```python
from build123d import *

# Parameters (mm, degrees)
EXTRUDE_1_DEPTH           = 20
FILLET_1_R                = 5
SKETCH_2_R                = 8
CUT_EXTRUDE_1_DEPTH       = 5
SKETCH_3_R                = 6
CUT_EXTRUDE_2_DEPTH       = 1
CUT_EXTRUDE_3_DEPTH       = 5
CUT_EXTRUDE_4_DEPTH       = 5
SKETCH_6_R                = 0.625
CUT_EXTRUDE_5_DEPTH       = 4
SKETCH_7_W                = 27
SKETCH_7_H                = 5
CUT_EXTRUDE_6_DEPTH       = 7
SKETCH_8_R                = 1.45
CUT_EXTRUDE_7_DEPTH       = 12
CUT_EXTRUDE_8_DEPTH       = 43.204857647
SKETCH_10_W               = 7.5
SKETCH_10_H               = 8.2
CUT_EXTRUDE_9_DEPTH       = 35.875672037
CUT_EXTRUDE_10_DEPTH      = 40.749968553
CUT_EXTRUDE_10_DEPTH_BACK = 40.749968553
SKETCH_11_R               = 1.455


with BuildPart() as part:
    # Эскиз1 → Бобышка-Вытянуть1 (new body)
    with BuildSketch(Plane(origin=(0, 0, 0), x_dir=(1, 0, 0), z_dir=(0, 1, 0))):
        Polygon((-13, 27.5), (-13, 0), (13, 0), (13, 27.5), (25, 27.5), (25, -7.5), (-25, -7.5), (-25, 27.5), align=None)
    extrude(amount=EXTRUDE_1_DEPTH)

    # Скругление1
    fillet_1_edges = [part.edges().sort_by_distance(p)[0] for p in [
        (19, 0, -27.5),
        (25, 10, -27.5),
        (-25, 10, -27.5),
        (-19, 20, -27.5),
        (-25, 20, -10),
        (25, 20, -10),
        (19, 20, -27.5),
        (25, 0, -10),
        (-25, 0, -10),
        (-19, 0, -27.5),
    ]]
    fillet(fillet_1_edges, radius=FILLET_1_R)

    # Эскиз2 → Вырез-Вытянуть1 (cut)
    with BuildSketch(Plane.ZY.offset(-13)):
        with Locations((-17.5, 10)):
            Circle(SKETCH_2_R)
    extrude(amount=-CUT_EXTRUDE_1_DEPTH, mode=Mode.SUBTRACT)

    # Эскиз3 → Вырез-Вытянуть2 (cut)
    with BuildSketch(Plane.ZY.offset(-18)):
        with Locations((-17.5, 10)):
            Circle(SKETCH_3_R)
    extrude(amount=-CUT_EXTRUDE_2_DEPTH, mode=Mode.SUBTRACT)

    # Эскиз4 → Вырез-Вытянуть3 (cut)
    with BuildSketch(Plane(origin=(-13, 0, 0), x_dir=(0, 0, -1), z_dir=(1, 0, 0))):
        with BuildLine():
            Line((13.195, 19.30212207), (2.9, 14.537620522))
            ThreePointArc((2.9, 14.537620522), (0, 10), (2.9, 5.462379478))
            Line((2.9, 5.462379478), (13.195, 0.69787793))
            ThreePointArc((13.195, 0.69787793), (27.75, 10), (13.195, 19.30212207))
        make_face()
    extrude(amount=-CUT_EXTRUDE_3_DEPTH, mode=Mode.SUBTRACT)

    # Эскиз5 → Вырез-Вытянуть4 (cut)
    with BuildSketch(Plane(origin=(-18, 0, 0), x_dir=(0, 0, -1), z_dir=(1, 0, 0))):
        with BuildLine():
            Line((19.4, 15.812916652), (19.4, 16.49838717))
            ThreePointArc((19.4, 16.49838717), (17.499999842, 18.39838717), (15.6, 16.498386854))
            Line((15.6, 16.498386854), (15.6, 15.665366642))
            ThreePointArc((15.6, 15.665366642), (15.094249889, 14.335999398), (13.832782732, 13.678959785))
            Line((13.832782732, 13.678959785), (1.932299859, 12.284367885))
            ThreePointArc((1.932299859, 12.284367885), (-0.1, 10), (1.932299859, 7.715632115))
            Line((1.932299859, 7.715632115), (13.832782732, 6.321040215))
            ThreePointArc((13.832782732, 6.321040215), (15.094249889, 5.664000602), (15.6, 4.334633358))
            Line((15.6, 4.334633358), (15.6, 3.501613146))
            ThreePointArc((15.6, 3.501613146), (17.5, 1.601613146), (19.4, 3.501613146))
            Line((19.4, 3.501613146), (19.4, 4.187083665))
            ThreePointArc((19.4, 4.187083665), (19.635266181, 5.128207436), (20.285714286, 5.847916677))
            ThreePointArc((20.285714286, 5.847916677), (22.5, 10), (20.285714286, 14.152083323))
            ThreePointArc((20.285714286, 14.152083323), (19.635266107, 14.871792704), (19.4, 15.812916652))
        make_face()
    extrude(amount=-CUT_EXTRUDE_4_DEPTH, mode=Mode.SUBTRACT)

    # Эскиз6 → Вырез-Вытянуть5 (cut)
    with BuildSketch(Plane(origin=(-23, 0, 0), x_dir=(0, 0, -1), z_dir=(1, 0, 0))):
        with Locations((2.278018202, 10)):
            Circle(SKETCH_6_R)
        with Locations((6.311115384, 10)):
            Circle(SKETCH_6_R)
        with Locations((10.428235425, 10)):
            Circle(SKETCH_6_R)
        with Locations((17.5, 14.907931149)):
            Circle(SKETCH_6_R)
        with Locations((17.5, 16.848859168)):
            Circle(SKETCH_6_R)
        with Locations((17.5, 5.082068851)):
            Circle(SKETCH_6_R)
        with Locations((17.5, 3.141140832)):
            Circle(SKETCH_6_R)
    extrude(amount=-CUT_EXTRUDE_5_DEPTH, mode=Mode.SUBTRACT)

    # Эскиз7 → Вырез-Вытянуть6 (cut)
    with BuildSketch(Plane.XY.offset(7.5)):
        with Locations((0, 17.5)):
            Rectangle(SKETCH_7_W, SKETCH_7_H)
        with Locations((0, 2.5)):
            Rectangle(SKETCH_7_W, SKETCH_7_H)
    extrude(amount=-CUT_EXTRUDE_6_DEPTH, mode=Mode.SUBTRACT)

    # Эскиз8 → Вырез-Вытянуть7 (cut)
    with BuildSketch(Plane(origin=(0, 15, 0), x_dir=(1, 0, 0), z_dir=(0, 1, 0))):
        with Locations(Location((-8.5, -4, 0), (0, 0, 270))):
            Circle(SKETCH_8_R)
        with Locations(Location((8.5, -4, 0), (0, 0, 270))):
            Circle(SKETCH_8_R)
    extrude(amount=-CUT_EXTRUDE_7_DEPTH, mode=Mode.SUBTRACT)

    # Эскиз9 → Вырез-Вытянуть8 (cut, through all)
    with BuildSketch(Plane.XZ):
        Polygon((13, 0), (17.25, 0), (17.25, 7.5), (-36.683406806, 12.049060371), (-29.579948377, -33.351304372), (-5.181112902, -33.351304372), (8.202214573, -2.26080516), align=None)
    extrude(amount=-CUT_EXTRUDE_8_DEPTH, mode=Mode.SUBTRACT)

    # Эскиз10 → Вырез-Вытянуть9 (cut, through all)
    with BuildSketch(Plane.ZY.offset(-17.25)):
        with Locations((3.75, 10)):
            Rectangle(SKETCH_10_W, SKETCH_10_H)
    extrude(amount=-CUT_EXTRUDE_9_DEPTH, mode=Mode.SUBTRACT)

    # Эскиз11 → Вырез-Вытянуть10 (cut, two sides: drawn at the far end of the back side and taken through both)
    with BuildSketch(Plane(origin=(0, 5.9, 0), x_dir=(1, 0, 0), z_dir=(0, 1, 0)).offset(-CUT_EXTRUDE_10_DEPTH_BACK)):
        with Locations(Location((21, -3.75, 0), (0, 0, 270))):
            Circle(SKETCH_11_R)
    extrude(amount=CUT_EXTRUDE_10_DEPTH + CUT_EXTRUDE_10_DEPTH_BACK, mode=Mode.SUBTRACT)


solid = part.part
```
Input: part model. Units: mm. Frame: model coordinates. A direction names the side the tool comes from. Round coordinates to 2 decimals unless told otherwise and drop trailing zeros. Order: outer loops, then holes, each group sorted by start corner. A loop starts at its lowest first (then second) coordinate and runs counter-clockwise, first axis right, second up. Notation, with made-up numbers: (0, 86.5) - (37, 86.5) arc R10 ccw to (37, 93.5) - close; hole circle Ø9 at (-1, 45). An arc over 180 degrees is marked (long way). Answer in a Markdown table with one row per item.
Item 1: Section query D-D (z = -17.5). Return the cut outline in (x, y).
Model answer:
| item | result |
|---|---|
| outline | (13, 0) - (20, 0) arc R5 ccw to (25, 5) - (25, 15) arc R5 ccw to (20, 20) - (13, 20) - (13, 18) - (18, 18) - (18, 16) - (19, 16) - (19, 4) - (18, 4) - (18, 2) - (13, 2) - close |
Item 2: Reachability of faces 1 (the flat face through (21, 5.9, 2)), 2 (the flat face through (18, 10, 0)), 3 (the flat face through (17.25, 3, 4)) from +Z, -Z, +X, -X, +Y, -Y: full face, straight path, thin tool, end or side. Return the list, or none.
Model answer:
| item | result |
|---|---|
| face 1 | +Z, +X, -X |
| face 2 | +Z, -X |
| face 3 | +Z, -X, +Y, -Y |
Item 3: Mould query, pull axis X, two halves, no side actions, for faces 4 (the cylindrical face through (19.58, 17.01, 3.43)), 5 (the cylindrical face through (16.55, 1.5, -26.07)), 6 (the flat face through (18, 16, -16)), 7 (the cylindrical face through (19.58, 2.91, 3.43)). Classes: released by +X, released by -X, zero draft, split by the parting line, or undercut.
Model answer:
| item | result |
|---|---|
| face 4 | undercut |
| face 5 | zero draft |
| face 6 | released by -X |
| face 7 | undercut |
Item 4: Section query A-A (x = 15). Return the cut outline in (y, z), then the cut area to 3 significant figures.
Model answer:
| item | result |
|---|---|
| outline | (0, -22.5) arc R5 ccw to (5, -27.5) - (15, -27.5) arc R5 ccw to (20, -22.5) - (20, 0) - (0, 0) - close; hole circle Ø16 at (10, -17.5) |
| area | 338 mm² |
Item 5: Section query C-C (y = 10). Return the cut outline in (x, z), then the cut area to 3 significant figures.
Model answer:
| item | result |
|---|---|
| outline | (13, -27.5) - (20, -27.5) arc R5 ccw to (25, -22.5) - (25, 0) - (13, 0) - (13, -9.5) - (18, -9.5) - (18, -11.5) - (19, -11.5) - (19, -23.5) - (18, -23.5) - (18, -25.5) - (13, -25.5) - close |
| area | 233 mm² |
Item 6: Pin query (flat end, axial travel): pin 1 (8 mm diameter, centred on y = 8, z = -16.5, fed in from -X); pin 2 (12 mm diameter, centred on y = 13.5, z = -22.5, fed in from -X); pin 3 (2 mm diameter, centred on y = 8, z = 1.5, fed in from -X); pin 4 (6 mm diameter, centred on x = 17, y = 9, fed in from +Z). Return the tip coordinate at first contact, or that it passes through.
Model answer:
| item | result |
|---|---|
| pin 1 | stops at x = 18 |
| pin 2 | stops at x = 13 |
| pin 3 | passes through |
| pin 4 | stops at z = 0 |
Item 7: Line query: line 1 (Y direction, x = 18.3, z = -17.5); line 2 (Y direction, x = 19, z = 2.5); line 3 (Z direction, x = 21, y = 4.3) (3 decimals). Output: solid intervals per line, ascending.
Model answer:
| item | result |
|---|---|
| line 1 | y = 0 to 4, 16 to 20 |
| line 2 | y = 0 to 5.9, 14.1 to 20 |
| line 3 | z = -27.349 to 2.295, 5.205 to 7.5 |
Item 8: Section query B-B (z = 3.75). Return the cut outline in (x, y) (3 decimals).
Model answer:
| item | result |
|---|---|
| outline | (17.25, 0) - (19.545, 0) - (19.545, 5.9) - (17.25, 5.9) - close; (17.25, 14.1) - (19.545, 14.1) - (19.545, 20) - (17.25, 20) - close; (22.455, 0.644) arc R5 ccw to (25, 5) - (25, 5.9) - (22.455, 5.9) - close; (22.455, 14.1) - (25, 14.1) - (25, 15) arc R5 ccw to (22.455, 19.356) - close |
